Study the drawing (mm; zero at the part's minimum x, y, z) and answer. Coordinates: 2 decimals unless noted, no trailing zeros. Loops run counter-clockwise (first coordinate to the right, second up) from the corner with the lowest first, then second, coordinate; pieces in that order, holes last. Notation, with made-up numbers: (-16.75, -32.75) - (12.25, -32.75) arc R20 ccw to (12.25, -1.75) - close; hole circle Ø10 at (-3.5, 32). An arc over 180 degrees is marked (long way). Use CSV: the item, a comma, the result in double quotes.
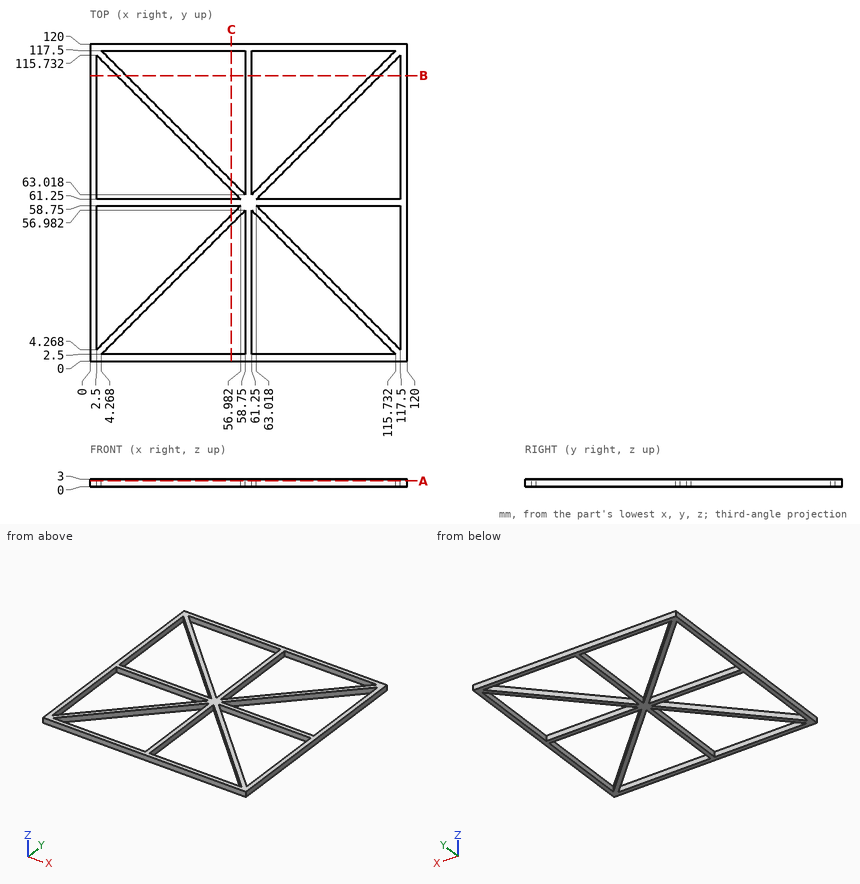
Q1. The part is cut by section C-C on x = 53.5. Determine the outline of the cut face in (y, z), and give its area (3 significant figures).
Reported:
outline,"(0, 0) - (2.5, 0) - (2.5, 3) - (0, 3) - close; (51.73, 0) - (55.27, 0) - (55.27, 3) - (51.73, 3) - close; (58.75, 0) - (61.25, 0) - (61.25, 3) - (58.75, 3) - close; (64.73, 0) - (68.27, 0) - (68.27, 3) - (64.73, 3) - close; (117.5, 0) - (120, 0) - (120, 3) - (117.5, 3) - close"
area,"43.7 mm²"
Q2. The part is cut by section B-B on y = 108. Determine the outline of the cut face in (x, z).
Reported:
outline,"(0, 0) - (2.5, 0) - (2.5, 3) - (0, 3) - close; (10.23, 0) - (13.77, 0) - (13.77, 3) - (10.23, 3) - close; (58.75, 0) - (61.25, 0) - (61.25, 3) - (58.75, 3) - close; (106.23, 0) - (109.77, 0) - (109.77, 3) - (106.23, 3) - close; (117.5, 0) - (120, 0) - (120, 3) - (117.5, 3) - close"
Q3. The part is cut by section A-A on z = 2.3. Give the number of separate pieces and of enclosed holes in the cut face, and give its area (3 significant figures).
Reported:
separate pieces,"1"
enclosed holes,"8"
area,"2,530 mm²"
Q4. Find the intervals of material crossed by probe 1 along X at (y, z) = (8.5, 2.2); probe 2 along X at (y, z) = (78.5, 1); probe 3 along Y at (x, z) = (103.5, 0.75), in increasing order. Write a range as [from, to].
Reported:
probe 1,"x = [0, 2.5], [6.73, 10.27], [58.75, 61.25], [109.73, 113.27], [117.5, 120]"
probe 2,"x = [0, 2.5], [39.73, 43.27], [58.75, 61.25], [76.73, 80.27], [117.5, 120]"
probe 3,"y = [0, 2.5], [14.73, 18.27], [58.75, 61.25], [101.73, 105.27], [117.5, 120]"
